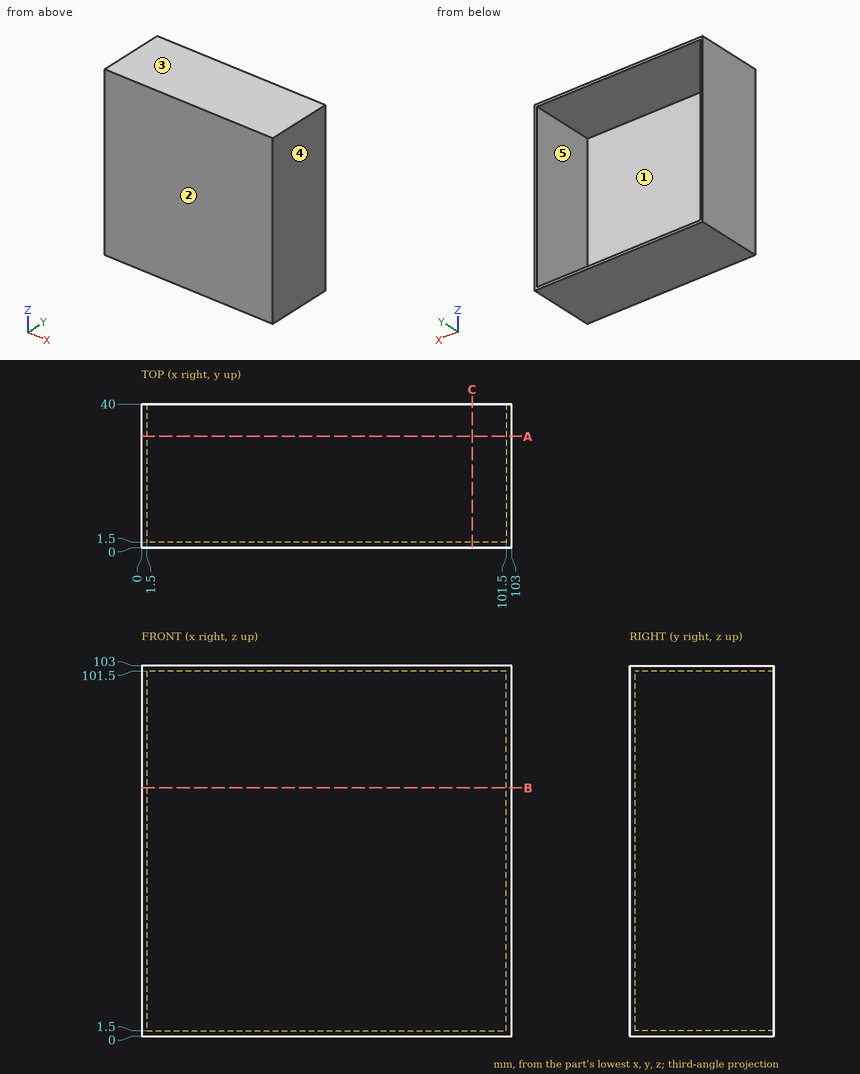
Verification items for this drawing (mm, ordinates from the low corner). A direction names the side the tool comes from. Coordinates: 2 decimals unless noted, no trailing zeros. Order: outer loops, then holes, each group sorted by start corner. A loop starts at its lowest first (then second) coordinate and runs counter-clockwise, first axis right, second up. Notation, with made-up numbers: (23, -7) -> (34, -7) arc R29 cw to (34, 32) -> close; hole circle Ø9 at (33, 10.25). An arc over 180 degrees is marked (long way). Put each result on its own line as item: value. Start each with the question number.
1. Go/stop test with flat-tipped pins: pin 1 Ø6 at (x, z) = (19.5, 41.5) entering from -Y; pin 2 Ø6 at (x, z) = (82, 47.5) entering from +Y. Record where each tip stops, or that it passes through.
2. Cross-section at C-C, the plane x = 92. Record the boundary of the cut face in (y, z).
3. Cross-section at A-A, the plane y = 31. Record the boundary of the cut face in (x, z).
4. Cross-section at B-B, the plane z = 69. Record the boundary of the cut face in (x, y), then the cut area to 3 significant figures.
5. Access from +Z, -Z, +X, -X, +Y, -Y to the whole of each face (thin tool, end or side, straight path). Record for the marked faces 4 and 5.
6. Mould release check, pull along Y, two halves, no side actions. Record for the marked faces 1, 2 and 3: released by +Y, released by -Y, zero draft, split by the parting line, or undercut.
7. Material ranges on L1, parallel to X at y = 11.5, z = 4.5; L2, parallel to Y at x = 84, z = 99, recorded low to high. Write a range as [from, to].
Computed:
1. pin 1: y = 0
1. pin 2: y = 1.5
2. outline: (0, 0) -> (40, 0) -> (40, 1.5) -> (1.5, 1.5) -> (1.5, 101.5) -> (40, 101.5) -> (40, 103) -> (0, 103) -> close
3. outline: (0, 0) -> (103, 0) -> (103, 103) -> (0, 103) -> close; hole (1.5, 1.5) -> (101.5, 1.5) -> (101.5, 101.5) -> (1.5, 101.5) -> close
4. outline: (0, 0) -> (103, 0) -> (103, 40) -> (101.5, 40) -> (101.5, 1.5) -> (1.5, 1.5) -> (1.5, 40) -> (0, 40) -> close
4. area: 270 mm2
5. face 4: +Z, -Z, +X, +Y, -Y
5. face 5: +Y
6. face 1: released by +Y
6. face 2: released by -Y
6. face 3: zero draft
7. L1: [0, 1.5], [101.5, 103]
7. L2: [0, 1.5]
